Work out the finished part from the listing and answer in its coordinate system (mm). Round coordinates to 2 decimals unless told otherwise and drop trailing zeros. Write each loop counter-clockwise with the first axis right and the second up, starting at its lowest first coordinate (ties: lowest second). Pieces come first, ordered by that corner, then holes. Notation, with made-up numbers: M 44.25,-27 L 83.25,-27 A27 cw 83.25,5 Z; hole C 5.5,-32 d8. An arc over 180 degrees is marked long. One line per item, written item: value. Start each with the question number.
Q1. Find section B-B (x = 40.5). Write down the section's boundary in (y, z).
Q2. Given pin 1 Ø8 at (x, y) = (13.5, 15.5) entering from -Z; pin 2 Ø1.5 at (y, z) = (-28.5, 1) entering from -X; pin 3 Ø1.5 at (x, z) = (33, 2) entering from -Y; pin 4 Ø1.5 at (x, z) = (-32, 1.5) entering from +Y, each flat-ended and moving along its own axis, determine where each tip first touches the part or whether it passes through.
Q3. Find section C-C (y = -20.5). Write down the section's boundary in (x, z), and give its area (3 significant figures).
Q4. Find section A-A (z = 1.15). Write down the section's boundary in (x, y), and give its area (3 significant figures).
Q5. Consider probe 1 along Y at (x, z) = (-36.5, 1.5); probe 2 along X at (y, z) = (-23, 0.65). Determine where each line is inside the solid, lowest interval first.
Autodesk Fusion 360 part; units mm, degrees
sketch "Sketch1" plane through (0, 0, 0) normal (0, 0, 1) x (1, 0, 0)
  line L0 (-46.5, 30) -> (46.5, 30)
  line L1 (46.5, 30) -> (46.5, -30)
  line L2 (46.5, -30) -> (-46.5, -30)
  line L3 (-46.5, -30) -> (-46.5, 30)
  line L4 (-46.5, 30) -> (46.5, -30) construction
  line L5 (46.5, 30) -> (-46.5, -30) construction
  line L6 (-46.5, 30) -> (-15.5, 30)
  line L7 (-15.5, 30) -> (-15.5, 27)
  line L8 (-15.5, 27) -> (-46.5, 27)
  line L9 (-46.5, 27) -> (-46.5, 30)
  line L10 (-46.5, -30) -> (-15.5, -30)
  line L11 (-15.5, -30) -> (-15.5, -27)
  line L12 (-15.5, -27) -> (-46.5, -27)
  line L13 (-46.5, -27) -> (-46.5, -30)
  line L14 (46.5, 30) -> (15.5, 30)
  line L15 (15.5, 30) -> (15.5, 27)
  line L16 (15.5, 27) -> (46.5, 27)
  line L17 (46.5, 27) -> (46.5, 30)
  line L18 (46.5, -30) -> (15.5, -30)
  line L19 (15.5, -30) -> (15.5, -27)
  line L20 (15.5, -27) -> (46.5, -27)
  line L21 (46.5, -27) -> (46.5, -30)
  line L22 (46.5, 30) -> (43.5, 30)
  line L23 (43.5, 30) -> (43.5, 27)
  line L24 (43.5, 27) -> (46.5, 27)
  line L25 (46.5, 27) -> (46.5, 30)
  line L26 (46.5, -30) -> (43.5, -30)
  line L27 (43.5, -30) -> (43.5, -27)
  line L28 (43.5, -27) -> (46.5, -27)
  line L29 (46.5, -27) -> (46.5, -30)
  line L30 (-46.5, 27) -> (-43.5, 27)
  line L31 (-43.5, 27) -> (-43.5, 9)
  line L32 (-43.5, 9) -> (-46.5, 9)
  line L33 (-46.5, 9) -> (-46.5, 27)
  line L34 (-46.5, -27) -> (-43.5, -27)
  line L35 (-43.5, -27) -> (-43.5, -9)
  line L36 (-43.5, -9) -> (-46.5, -9)
  line L37 (-46.5, -9) -> (-46.5, -27)
  dimension "d1" = 93
  dimension "d2" = 60
  dimension "d3" = 31
  dimension "d4" = 3
  dimension "d5" = 31
  dimension "d6" = 3
  dimension "d7" = 31
  dimension "d8" = 3
  dimension "d9" = 31
  dimension "d10" = 3
  dimension "d11" = 3
  dimension "d12" = 3
  dimension "d13" = 3
  dimension "d14" = 3
  dimension "d15" = 3
  dimension "d16" = 18
  dimension "d17" = 3
  dimension "d18" = 18
extrude "Extrude1" add sketch "Sketch1" along normal blind 3 contours L0 L1 L2 L3 L7 L8 L11 L12 L15 L16 L19 L20 L24 L28 L31 L32 L35 L36
sketch "Sketch2" plane through (0, 0, 3) normal (0, 0, 1) x (-1, 0, 0)
  line L0 (-15.5, 30) -> (-15.5, 27)
  line L1 (-15.5, 27) -> (-46.5, 27)
  line L2 (-46.5, 27) -> (-46.5, -27)
  line L3 (-46.5, -27) -> (-15.5, -27)
  line L4 (-15.5, -27) -> (-15.5, -30)
  line L5 (-15.5, -30) -> (15.5, -30)
  line L6 (15.5, -30) -> (15.5, -27)
  line L7 (15.5, -27) -> (43.5, -27)
  line L8 (43.5, -27) -> (43.5, -9)
  line L9 (43.5, -9) -> (46.5, -9)
  line L10 (46.5, -9) -> (46.5, 9)
  line L11 (46.5, 9) -> (43.5, 9)
  line L12 (43.5, 9) -> (43.5, 27)
  line L13 (43.5, 27) -> (15.5, 27)
  line L14 (15.5, 27) -> (15.5, 30)
  line L15 (15.5, 30) -> (-15.5, 30)
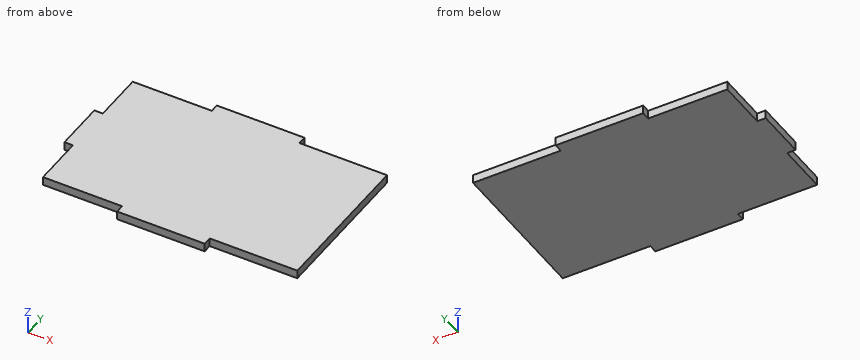
The answers:
1. outline: M -27,0 L 27,0 L 27,3 L -27,3 Z
2. pin 1: z = 0
2. pin 2: x = -15.5
2. pin 3: y = -27
2. pin 4: y = 27
3. outline: M -43.5,0 L 46.5,0 L 46.5,3 L -43.5,3 Z
3. area: 270 mm2
4. outline: M -46.5,-9 L -43.5,-9 L -43.5,-27 L -15.5,-27 L -15.5,-30 L 15.5,-30 L 15.5,-27 L 46.5,-27 L 46.5,27 L 15.5,27 L 15.5,30 L -15.5,30 L -15.5,27 L -43.5,27 L -43.5,9 L -46.5,9 Z
4. area: 5,100 mm2
5. probe 1: -27 to 27
5. probe 2: -43.5 to 46.5
